Here's how the part is built. I have some questions about the finished solid (model axes, mm). Face numbers are marked on the shaded views. Give positions to 0.01 mm unless a question says otherwise; leave off trailing zeros. Loops run counter-clockwise (first coordinate to the right, second up) from the corner with the lowest first, then second, coordinate; pieces in that order, holes last. Notation, with made-up numbers: (-19, 74) - (-9, 74) arc R33 cw to (-9, 109) - close; hole circle Ø2 at (-31.75, -4.75). An arc over 180 degrees is marked (long way). One line per item, written item: value. Start each with the question number.
```python
from build123d import *

# Parameters (mm, degrees)
F0_W          = 431.8
F0_H          = 88.9
F1_DEPTH      = 279.4
F2_R          = 63.5
F3_DEPTH      = 127
F5_DEPTH      = 227.33
F5_DEPTH_BACK = 269.24


with BuildPart() as f1:
    # F0 (on Front) → F1 (new body)
    with BuildSketch(Plane.XZ):
        Rectangle(F0_W, F0_H)
    extrude(amount=-F1_DEPTH)

    # F2 (on face) → F3 (cut)
    with BuildSketch(Plane.XY.offset(44.45)):
        with Locations((-196.85, 53.975)):
            Circle(F2_R)
        with Locations((196.85, 53.975)):
            Circle(F2_R)
    extrude(amount=-F3_DEPTH, mode=Mode.SUBTRACT)

    # F4 (on Right) → F5 (cut, two sides)
    with BuildSketch(Plane.YZ) as f5_sk:
        Polygon((0, 44.45), (0, 27.305), (53.975, 44.45), align=None)
        Polygon((0, -44.45), (53.975, -44.45), (0, -27.305), align=None)
    extrude(amount=-F5_DEPTH, mode=Mode.SUBTRACT)
    extrude(f5_sk.sketch, amount=F5_DEPTH_BACK, mode=Mode.SUBTRACT)


solid = f1.part
```
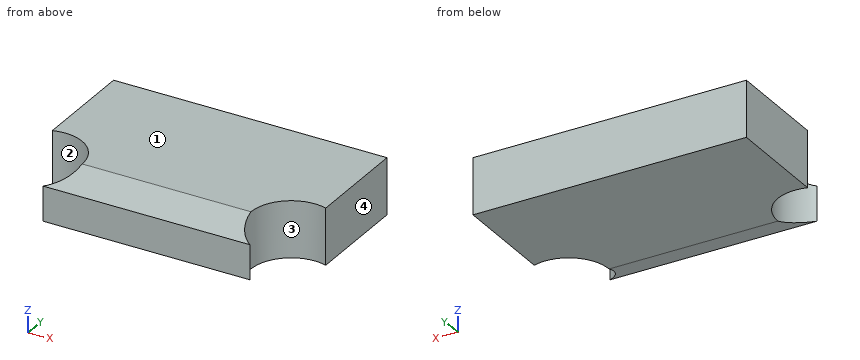
(1) If we section it at C-C on z = -12.5: List the corners of the cut face in (x, y) for me (3 decimals), plus the area to 3 significant figures.
(2) Will these pins go through, and if not, where does the flat tip stop? pin 1 (8 mm diameter, centred on x = 54, y = 47.5, fed in from -Z); pin 2 (4 mm diameter, centred on y = 29, z = 17.5, fed in from -X); pin 3 (12 mm diameter, centred on x = -21.5, y = 43.5, fed in from +Z).
(3) Please list where these lines run through material, in increasing order: probe 1 along X at (y, z) = (108, 19.5); probe 2 along Z at (x, y) = (42, 18.5); probe 3 along X at (y, z) = (73, 11). Write a range as from..to.
(4) If we mould it in two halves opening along X, with no side actions, what happens to the marked faces 1, 2, 3 and 4? For each: pulls with the +X half, pulls with the -X half, needs draft (parallel to the pull), parting line crosses it, or undercut.
(5) If we section it at D-D on y = 88: List the corners of the cut face in (x, z) for me, plus the area to 3 significant figures.
(6) If we section it at B-B on x = -62: List the corners of the cut face in (y, z) for me (3 decimals), plus the area to 3 significant figures.
(7) If we section it at A-A on x = -140: List the corners of the cut face in (y, z) for me (3 decimals).
Found:
1. outline: (-215.9, 114.55) arc R63.5 cw to (-163.399, 0) - (163.399, 0) arc R63.5 cw to (215.9, 114.55) - (215.9, 279.4) - (-215.9, 279.4) - close
1. area: 104,000 mm^2
2. pin 1: z = -43.66
2. pin 2: x = -139.36
2. pin 3: z = 43.03
3. probe 1: -163.48..163.48
3. probe 2: -33.18..33.18
3. probe 3: -136.27..136.27
4. face 1: needs draft
4. face 2: undercut
4. face 3: undercut
4. face 4: pulls with the +X half
5. outline: (-143.24, -44.45) - (143.24, -44.45) - (143.24, 44.45) - (-143.24, 44.45) - close
5. area: 25,500 mm^2
6. outline: (0, -27.305) - (53.975, -44.45) - (279.4, -44.45) - (279.4, 44.45) - (53.975, 44.45) - (0, 27.305) - close
6. area: 23,900 mm^2
7. outline: (0, -27.305) - (25.685, -35.464) - (25.685, 35.464) - (0, 27.305) - close; (82.265, -44.45) - (279.4, -44.45) - (279.4, 44.45) - (82.265, 44.45) - close
